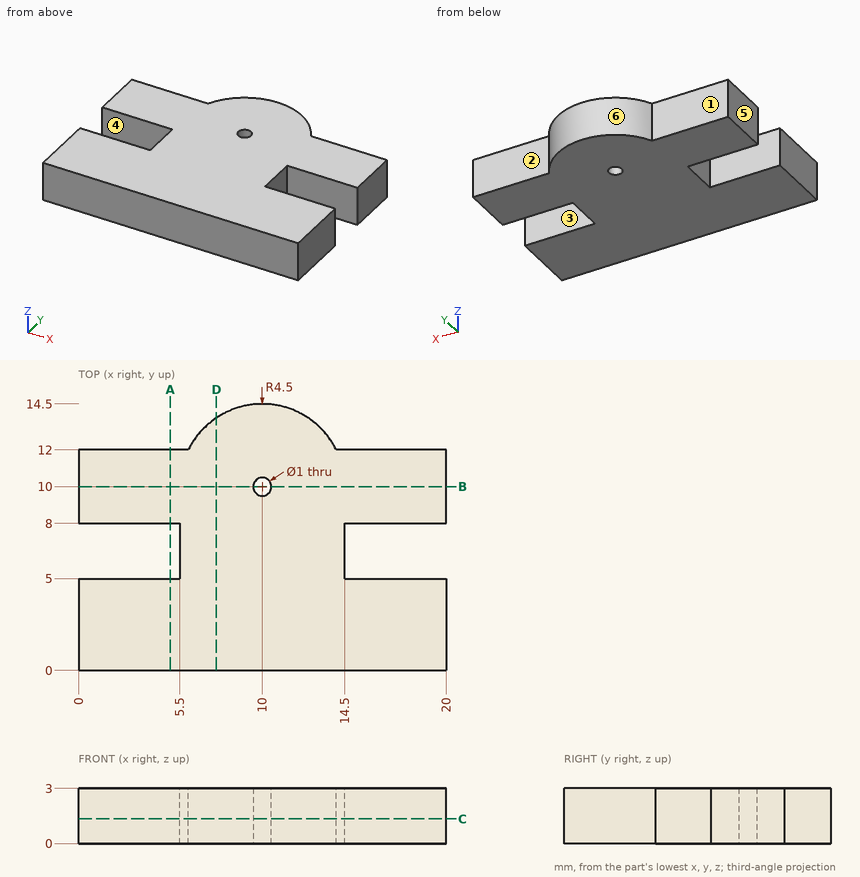
Print and shaded views of the part. All mm, measured from the part's lowest x, y and z. A direction names the side the tool comes from. Round coordinates to 2 decimals unless told otherwise and drop trailing zeros. Write each loop counter-clockwise with the first axis right and the second up, starting at its lowest first coordinate (ties: lowest second). Pieces come first, ordered by that corner, then holes. Notation, with made-up numbers: (-15.75, -2) - (6.25, -2) arc R16 ccw to (6.25, 29) - close; hole circle Ø8 at (1, 60.5). An arc over 180 degrees is marked (long way). Write each question's results on one line, items separated by ' | '. Start each with the question number.
Item 1: Mould opens along Y. For the marked faces 4, 5 and 6 say: pulls with the +Y half, pulls with the -Y half, needs draft (parallel to the pull), parting line crosses it, or undercut.
Item 2: Wall check: L1, parallel to X at y = 10, z = 1.4; L2, parallel to Y at x = 15.75, z = 0.1; L3, parallel to Y at x = 10, z = 1.4. Give the ranges that are in metal, low to high. Write a range as [from, to].
Item 3: Saw through at A-A (x = 5). Write the cut outline in (y, z).
Item 4: Drop flat-ended pins along their axis: P1, Ø1, axis at x = 15.5, z = 1.5, coming from the +Y side; P2, Ø1.5, axis at y = 7, z = 2, coming from the +X side. Give the stop position or say it passes through.
Item 5: Which spindle directions (+Z, -Z, +X, -X, +Y, -Y) get a long thin tool onto all of the face, cutting with end or side? Do the marked faces 1, 2 and 3. Say none if no direction does.
Item 6: Saw through at C-C (z = 1.35). Write the cut outline in (x, y).
Item 7: Saw through at D-D (x = 7.5). Write the cut outline in (y, z), and give its area (3 significant figures).
Item 8: Saw through at B-B (y = 10). Write the cut outline in (x, z).
Results are:
1) face 4: undercut | face 5: needs draft | face 6: pulls with the +Y half
2) L1: x = [0, 9.5], [10.5, 20] | L2: y = [0, 5], [8, 12] | L3: y = [0, 9.5], [10.5, 14.5]
3) outline: (0, 0) - (5, 0) - (5, 3) - (0, 3) - close; (8, 0) - (12, 0) - (12, 3) - (8, 3) - close
4) P1: stops at y = 12 | P2: stops at x = 14.5
5) face 1: +Z, -Z, -X, +Y | face 2: +Z, -Z, +X, +Y | face 3: +Z, -Z, +X
6) outline: (0, 0) - (20, 0) - (20, 5) - (14.5, 5) - (14.5, 8) - (20, 8) - (20, 12) - (14.03, 12) arc R4.5 ccw to (5.97, 12) - (0, 12) - (0, 8) - (5.5, 8) - (5.5, 5) - (0, 5) - close; hole circle Ø1 at (10, 10)
7) outline: (0, 0) - (13.74, 0) - (13.74, 3) - (0, 3) - close | area: 41.2 mm²
8) outline: (0, 0) - (9.5, 0) - (9.5, 3) - (0, 3) - close; (10.5, 0) - (20, 0) - (20, 3) - (10.5, 3) - close
